from build123d import *

# Parameters (mm, degrees)
SKETCH_1_W              = 23
SKETCH_1_H              = 13
EXTRUDE_1_DEPTH         = 10
EXTRUDE_START           = 10
SKETCH_1_5_W            = 4
SKETCH_1_5_H            = 22
SKETCH_1_5_W_2          = 5
SKETCH_1_5_H_2          = 20
EXTRUDE_2_DEPTH         = 5
SKETCH_9_R              = 21.75
SKETCH_9_R_2            = 18.75
SKETCH_9_R_3            = 8
EXTRUDE_4_DEPTH         = 6
SKETCH_9_5_R            = 18.75
CUT_EXTRUDE_4_DEPTH     = 4
FILLET_6_R              = 1
SKETCH_10_R             = 1
CUT_EXTRUDE_5_DEPTH     = 4
FILLET_3_R              = 1
HOLE_WIZARD_M1_41_D     = 1.6
HOLE_WIZARD_M1_41_DEPTH = 4.519311505
HOLE_WIZARD_M1_41_TIP   = 0.480688495
FILLET_7_R              = 3
FILLET_8_R              = 16


with BuildPart() as part:
    # Эскиз1 → Бобышка-Вытянуть1 (new body)
    with BuildSketch(Plane.XY):
        Polygon((-17, -11), (21, -11), (21, 11), (-17, 11), (-19, 10), (-24, 10), (-24, -10), (-19, -10), align=None)
        Rectangle(SKETCH_1_W, SKETCH_1_H, mode=Mode.SUBTRACT)
    extrude(amount=EXTRUDE_1_DEPTH)

    # Эскиз1<5> → Бобышка-Вытянуть2 (add)
    with BuildSketch(Plane.XY.offset(EXTRUDE_START)):
        Polygon((-11.5, 6.5), (11.5, 6.5), (17, 6.5), (17, 11), (-17, 11), (-17, 6.5), align=None)
        with Locations((19, 0)):
            Rectangle(SKETCH_1_5_W, SKETCH_1_5_H)
        Polygon((17, -6.5), (11.5, -6.5), (-11.5, -6.5), (-17, -6.5), (-17, -11), (17, -11), align=None)
        Polygon((-19, -10), (-19, 10), (-17, 11), (-17, -11), align=None)
        with Locations((-21.5, 0)):
            Rectangle(SKETCH_1_5_W_2, SKETCH_1_5_H_2)
    extrude(amount=EXTRUDE_2_DEPTH)

    # Эскиз9 → Бобышка-Вытянуть4 (add)
    # profile 1 of 3: a face of its own
    with BuildSketch(Plane.ZY.offset(24)):
        with Locations((-32.7, 0)):
            Circle(SKETCH_9_R)
        with Locations((-32.7, 0)):
            Circle(SKETCH_9_R_2, mode=Mode.SUBTRACT)
    # profile 2 of 3: a face of its own
    with BuildSketch(Plane.ZY.offset(24)):
        with BuildLine():
            ThreePointArc((-10.95, 0), (-14.616118395, -12.08452424), (-24.378572515, -20.095182124))
            Line((-24.378572515, -20.095182124), (0, -10))
            Line((0, -10), (0, 10))
            Line((0, 10), (-24.378572515, 20.095182124))
            ThreePointArc((-24.378572515, 20.095182124), (-14.616118395, 12.08452424), (-10.95, 0))
        make_face()
    # profile 3 of 3: a face of its own
    with BuildSketch(Plane.ZY.offset(24)):
        with Locations((-32.7, 0)):
            Circle(SKETCH_9_R_2)
        with Locations((-32.7, 0)):
            Circle(SKETCH_9_R_3, mode=Mode.SUBTRACT)
    extrude(amount=-EXTRUDE_4_DEPTH)

    # Эскиз9<5> → Вырез-Вытянуть4 (cut)
    with BuildSketch(Plane.ZY.offset(24)):
        with Locations((-32.7, 0)):
            Circle(SKETCH_9_5_R)
    extrude(amount=-CUT_EXTRUDE_4_DEPTH, mode=Mode.SUBTRACT)

    # Скругление6
    fillet_6_edges = [part.edges().sort_by_distance(p)[0] for p in [
        (-24, 0, -51.45),
        (-24, 0, -54.45),
        (-24, -15.047591062, -12.189286258),
        (-24, 15.047591062, -12.189286258),
    ]]
    fillet(fillet_6_edges, radius=FILLET_6_R)

    # Эскиз10 → Вырез-Вытянуть5 (cut)
    with BuildSketch(Plane.ZY.offset(20)):
        with Locations((-45.698540936, 0)):
            Circle(SKETCH_10_R)
        with Locations((-39.198031114, 11.257782204)):
            Circle(SKETCH_10_R)
        with Locations((-26.198250825, 11.257066663)):
            Circle(SKETCH_10_R)
        with Locations((-19.698980357, -0.001431082)):
            Circle(SKETCH_10_R)
        with Locations((-26.199490179, -11.259213286)):
            Circle(SKETCH_10_R)
        with Locations((-39.199270468, -11.258497745)):
            Circle(SKETCH_10_R)
    extrude(amount=-CUT_EXTRUDE_5_DEPTH, mode=Mode.SUBTRACT)

    # Скругление3
    fillet_3_edges = [part.edges().sort_by_distance(p)[0] for p in [
        (0, 6.5, 15),
        (17, 0, 15),
        (-17, 0, 15),
        (0, -6.5, 15),
    ]]
    fillet(fillet_3_edges, radius=FILLET_3_R)

    # Отверстие с зазором M1.41
    with Locations(Plane.XY.offset(10)):
        with Locations((13.85, 0), (-13.85, 0)):
            Hole(HOLE_WIZARD_M1_41_D / 2, depth=HOLE_WIZARD_M1_41_DEPTH)
            with Locations((0, 0, -(HOLE_WIZARD_M1_41_DEPTH + HOLE_WIZARD_M1_41_TIP / 2))):  # 118° drill point
                Cone(0, HOLE_WIZARD_M1_41_D / 2, HOLE_WIZARD_M1_41_TIP, mode=Mode.SUBTRACT)

    # Скругление7
    # the kernel refuses this fillet: 3 mm, written as the material it takes off along each edge
    with BuildSketch(Plane(origin=(18, -8, 12), x_dir=(0, -1, 0), z_dir=(0, 0, 1))) as fillet_7_piece_1_section:
        Polygon((0, 0), (FILLET_7_R, 0), (FILLET_7_R, FILLET_7_R), (0, FILLET_7_R), align=None)
    fillet_7_piece_1 = extrude(amount=FILLET_7_R, mode=Mode.PRIVATE)
    fillet_7_piece_1 = fillet_7_piece_1 - Plane(origin=(18, -8, 12), x_dir=(-0.7071067811865475, 0.7071067811865475, 0), z_dir=(0, 0, 1)) * Sphere(FILLET_7_R, mode=Mode.PRIVATE)
    add(fillet_7_piece_1, mode=Mode.SUBTRACT)
    with BuildSketch(Plane(origin=(18, 8, 12), x_dir=(1, 0, 0), z_dir=(0, 0, 1))) as fillet_7_piece_2_section:
        Polygon((0, 0), (FILLET_7_R, 0), (FILLET_7_R, FILLET_7_R), (0, FILLET_7_R), align=None)
    fillet_7_piece_2 = extrude(amount=FILLET_7_R, mode=Mode.PRIVATE)
    fillet_7_piece_2 = fillet_7_piece_2 - Plane(origin=(18, 8, 12), x_dir=(-0.7071067811865475, -0.7071067811865476, 0), z_dir=(0, 0, 1)) * Sphere(FILLET_7_R, mode=Mode.PRIVATE)
    add(fillet_7_piece_2, mode=Mode.SUBTRACT)
    with BuildSketch(Plane(origin=(21, -8, 15), x_dir=(-1, 0, 0), z_dir=(0, 1, 0))) as fillet_7_piece_3:
        with BuildLine():
            CenterArc((FILLET_7_R, -FILLET_7_R), FILLET_7_R, 90, 90)
            Line((0, -FILLET_7_R), (0, 0))
            Line((0, 0), (FILLET_7_R, 0))
        make_face()
    extrude(amount=16, mode=Mode.SUBTRACT)
    with BuildSketch(Plane(origin=(-24.5, -11, 15), x_dir=(0, 1, 0), z_dir=(1, 0, 0)), Plane(origin=(18, 11, 15), x_dir=(0, -1, 0), z_dir=(-1, 0, 0))) as fillet_7_piece_4:
        with BuildLine():
            CenterArc((FILLET_7_R, -FILLET_7_R), FILLET_7_R, 90, 90)
            Line((0, -FILLET_7_R), (0, 0))
            Line((0, 0), (FILLET_7_R, 0))
        make_face()
    extrude(amount=42.5, mode=Mode.SUBTRACT)
    with BuildSketch(Plane(origin=(21, 11, -7.5), x_dir=(0, -1, 0), z_dir=(0, 0, 1)), Plane(origin=(21, -11, -7.5), x_dir=(-1, 0, 0), z_dir=(0, 0, 1))) as fillet_7_piece_5:
        with BuildLine():
            CenterArc((FILLET_7_R, -FILLET_7_R), FILLET_7_R, 90, 90)
            Line((0, -FILLET_7_R), (0, 0))
            Line((0, 0), (FILLET_7_R, 0))
        make_face()
    extrude(amount=19.5, mode=Mode.SUBTRACT)
    with BuildSketch(Plane(origin=(-24, -17.5, 15), x_dir=(1, 0, 0), z_dir=(0, 1, 0))) as fillet_7_piece_6:
        with BuildLine():
            CenterArc((FILLET_7_R, FILLET_7_R), FILLET_7_R, 180, 90)
            Line((0, FILLET_7_R), (0, 0))
            Line((0, 0), (FILLET_7_R, 0))
        make_face()
    extrude(amount=35, mode=Mode.SUBTRACT)

    # Скругление8
    # the kernel refuses this fillet: 16 mm, written as the material it adds along each edge
    with BuildSketch(Plane(origin=(-18, -50, 0), x_dir=(1, 0, 0), z_dir=(0, 1, 0))) as fillet_8_piece_1_section:
        with BuildLine():
            CenterArc((FILLET_8_R, FILLET_8_R), FILLET_8_R, 180, 90)
            Line((0, FILLET_8_R), (0, 0))
            Line((0, 0), (FILLET_8_R, 0))
        make_face()
    fillet_8_piece_1 = extrude(amount=100, mode=Mode.PRIVATE)
    fillet_8_piece_1 = split(fillet_8_piece_1, bisect_by=Plane(origin=(-17.157282296, -13.337247559, -8.059025643), z_dir=(0, 0.9239164195137738, -0.38259436712117)), keep=Keep.TOP, mode=Mode.PRIVATE)
    fillet_8_piece_1 = split(fillet_8_piece_1, bisect_by=Plane(origin=(-17.157282296, 9.732934462, 0.644929087), z_dir=(0, -0.9239164195137736, -0.3825943671211702)), keep=Keep.TOP, mode=Mode.PRIVATE)
    fillet_8_piece_1 = split(fillet_8_piece_1, bisect_by=Plane(origin=(-11.5, -12.311624775, -8.483736679), z_dir=(-1, 0, 0)), keep=Keep.TOP, mode=Mode.PRIVATE)
    add(fillet_8_piece_1)
    with BuildSketch(Plane(origin=(-18, -50, 0), x_dir=(1, 0, 0), z_dir=(0, 1, 0))) as fillet_8_piece_2_section:
        with BuildLine():
            CenterArc((FILLET_8_R, FILLET_8_R), FILLET_8_R, 180, 90)
            Line((0, FILLET_8_R), (0, 0))
            Line((0, 0), (FILLET_8_R, 0))
        make_face()
    fillet_8_piece_2 = extrude(amount=100, mode=Mode.PRIVATE)
    fillet_8_piece_2 = split(fillet_8_piece_2, bisect_by=Plane(origin=(-11.244845554, -6.5, -2.767260165), z_dir=(0, -1, 0)), keep=Keep.TOP, mode=Mode.PRIVATE)
    fillet_8_piece_2 = split(fillet_8_piece_2, bisect_by=Plane(origin=(-11.244845554, -11.135244088, -2.741469147), z_dir=(0, 0.9239164195137738, -0.38259436712117)), keep=Keep.TOP, mode=Mode.PRIVATE)
    add(fillet_8_piece_2)
    with BuildSketch(Plane(origin=(-18, -50, 0), x_dir=(1, 0, 0), z_dir=(0, 1, 0))) as fillet_8_piece_3_section:
        with BuildLine():
            CenterArc((FILLET_8_R, FILLET_8_R), FILLET_8_R, 180, 90)
            Line((0, FILLET_8_R), (0, 0))
            Line((0, 0), (FILLET_8_R, 0))
        make_face()
    fillet_8_piece_3 = extrude(amount=100, mode=Mode.PRIVATE)
    fillet_8_piece_3 = split(fillet_8_piece_3, bisect_by=Plane(origin=(-9.25068262, 6.5, -0.972078171), z_dir=(0, 1, 0)), keep=Keep.TOP, mode=Mode.PRIVATE)
    fillet_8_piece_3 = split(fillet_8_piece_3, bisect_by=Plane(origin=(-9.25068262, 10.116600815, -0.281576041), z_dir=(0, -0.9239164195137736, -0.3825943671211702)), keep=Keep.TOP, mode=Mode.PRIVATE)
    add(fillet_8_piece_3)


solid = part.part
Could you check a few things on this model? Use its own coordinates, in mm. A direction names the side the tool comes from. Round coordinates to 2 decimals unless told otherwise and drop trailing zeros. Write each loop counter-clockwise with the first axis right and the second up, starting at its lowest first coordinate (ties: lowest second). Pieces come first, ordered by that corner, then holes. Notation, with made-up numbers: (-15, -2) - (44, -2) arc R18 cw to (44, 19) - close; hole circle Ø10 at (85.5, 45). An arc over 180 degrees is marked (long way). Put each result on its own line as item: value. Start each with the question number.
(1) Thinking about a two-plate mould opening in Z: for faces 1 (the flat face through (-18, -5, -40)), 2 (the conical face through (-13.72, 0.04, 5.08)), 3 (the cylindrical face through (-19.014, 11.558, -38.244)), which applies, released by +Z, released by -Z, zero draft, split by the parting line, or undercut?
(2) I want a section at B-B, the plane z = -32.7. Please give me the cut outline in (x, y).
(3) I want a section at C-C, the plane x = 16. Please give me the cut outline in (y, z).
(4) I want a section at A-A, the plane x = 3.5. Please give me the cut outline in (y, z), plus the area to 3 significant figures.
(5) Will these pins go through, and if not, where does the flat tip stop? pin 1 (1.2 mm diameter, centred on y = 1.5, z = 12.5, fed in from +X); pin 2 (10 mm diameter, centred on y = -10.5, z = -29, fed in from -X); pin 3 (1.5 mm diameter, centred on x = -22.5, z = 3, fed in from +Y); pin 4 (3 mm diameter, centred on x = -18.5, z = -41, fed in from -Y).
(6) I want a section at D-D, the plane y = -5.5. Give the number of separate pieces and of enclosed holes in the cut face, plus the area to 3 significant figures.
(7) For faces 4 (the cylindrical face through (-21.521, 5.632, -14.816)), 5 (the flat face through (11.5, 0, 5)), 6 (the flat face through (1, 11, 6)), 7 (the flat face through (-22, 10, 6)), 8 (the flat face through (-17, 0, 12)), which set-ups out of +Z, -Z, +X, -X, +Y, -Y let a thin tool reach every point of the face, with its end or its side?
(8) I need wall thicknesses on probe 1 along X at (y, z) = (0, 8); probe 2 along Y at (x, z) = (7, 2); probe 3 along Y at (x, z) = (13.85, 9). Which ranges of each line are inside material? Lowest first, please.
Here are the results:
1. face 1: zero draft
1. face 2: released by +Z
1. face 3: undercut
2. outline: (-24, -20.75) arc R1 ccw to (-23, -21.75) - (-18, -21.75) - (-18, -8) - (-20, -8) - (-20, -18.75) - (-23, -18.75) arc R1 ccw to (-24, -19.75) - close; (-24, 19.75) arc R1 ccw to (-23, 18.75) - (-20, 18.75) - (-20, 8) - (-18, 8) - (-18, 21.75) - (-23, 21.75) arc R1 ccw to (-24, 20.75) - close
3. outline: (-11, 0) - (11, 0) - (11, 12) arc R3 ccw to (8, 15) - (7.5, 15) arc R1 ccw to (6.5, 14) - (6.5, 10) - (-6.5, 10) - (-6.5, 14) arc R1 ccw to (-7.5, 15) - (-8, 15) arc R3 ccw to (-11, 12) - close
4. outline: (-11, 0) - (-6.5, 0) - (-6.5, 14) arc R1 ccw to (-7.5, 15) - (-8, 15) arc R3 ccw to (-11, 12) - close; (6.5, 0) - (11, 0) - (11, 12) arc R3 ccw to (8, 15) - (7.5, 15) arc R1 ccw to (6.5, 14) - close
4. area: 131 mm^2
5. pin 1: stops at x = 21
5. pin 2: stops at x = -20
5. pin 3: stops at y = 10
5. pin 4: stops at y = -20.66
6. separate pieces: 3
6. enclosed holes: 0
6. area: 471 mm^2
7. face 4: -X
7. face 5: +Z, -Z
7. face 6: +Z, +X, -X, +Y
7. face 7: +Z, -X, +Y
7. face 8: +Z
8. probe 1: x = -24 to -14.65, -13.05 to -11.5, 11.5 to 13.05, 14.65 to 21
8. probe 2: y = -11 to -6.5, 6.5 to 11
8. probe 3: y = -11 to -0.8, 0.8 to 11
